Design review of the part built by this model. Coordinates are the model's own, in mm. A direction names the side the tool comes from. Coordinates: 2 decimals unless noted, no trailing zeros. Write each loop counter-clockwise with the first axis right and the second up, starting at its lowest first coordinate (ties: lowest second). Pieces come first, ordered by that corner, then holes. Notation, with made-up numbers: (52, 75.5) - (107, 75.5) arc R21 cw to (107, 109.5) - close; hole circle Ø11 at (-16, 52). An arc over 180 degrees is marked (long way). Answer as CSV lines item,"result". Start each with the question number.
Q1. Machinability: for faces 1 (the face through (0.54, -8.88, -11.56)), 2 (the face through (0.75, -66, 0)), 3 (the face through (4, -70, 0)), 4 (the face through (-1, -42, -12)), 5 (the face through (0, -20, 19)), which of the approach directions +Z, -Z, +X, -X, +Y, -Y give a long, thin tool a straight path to every point of the face, cutting with its end or side? Answer none if there is none.
Q2. We need section C-C (y = -51.5). Write out the cut boundary in (x, z).
Q3. For line 1 along Z through (x, y) = (0, -12.5); line 2 along X through (y, z) = (-4.75, 14); line 3 along Z through (x, y) = (0.5, -12.5), list the stretches that pass through material, from the lowest coordinate up. Write a range as [from, to].
Q4. Mouldability with a two-part tool opening along X and no side actions: class faces 6 (the face through (-1, -42, 12)), 7 (the face through (1.65, -69.14, -0.17)), 8 (the face through (0.23, -18.24, -14.37)) as pulls with the +X half, pulls with the -X half, needs draft (parallel to the pull), parting line crosses it, or undercut.
Q5. We need section A-A (y = -15). Write out the cut boundary in (x, z), plus the area to 3 significant figures.
Q6. Clearance check with flat-ended pins moving along their axes: pin 1 (1 mm diameter, centred on x = 4, z = 3.5, fed in from +Y); pin 2 (6 mm diameter, centred on x = 0, z = 14, fed in from -Y); pin 3 (5.5 mm diameter, centred on x = -0.5, z = -20, fed in from -Y); pin 4 (0.6 mm diameter, centred on y = -66.5, z = -2, fed in from -X). State where each tip first meets the part, or that it passes through.
Q7. We need section D-D (y = -62). Write out the cut boundary in (x, z).
Q8. We need section B-B (z = 8.5). Write out the cut boundary in (x, y).
from build123d import *

# Parameters (mm, degrees)
SKETCH1_W                   = 10.5
SKETCH1_H                   = 24
BOSS_EXTRUDE1_DEPTH         = 70
CUT_EXTRUDE1_REACH          = 76.186
FILLET1_R                   = 3
SKETCH3_W                   = 10.5
SKETCH3_H                   = 44
BOSS_EXTRUDE2_DEPTH         = 20
FILLET2_R                   = 1
M6_TAPPED_HOLE1_D           = 5
M6_TAPPED_HOLE1_DEPTH       = 17
M6_TAPPED_HOLE1_CSINK_D     = 6.05
M6_TAPPED_HOLE1_CSINK_ANGLE = 90
M6_TAPPED_HOLE1_TIP         = 1.502151548
FILLET3_R                   = 5
FILLET4_R                   = 1


with BuildPart() as part:
    # Sketch1 → Boss-Extrude1 (new body)
    with BuildSketch(Plane(origin=(0, 0, 0), x_dir=(1, 0, 0), z_dir=(0, 1, 0))):
        Rectangle(SKETCH1_W, SKETCH1_H)
    extrude(amount=-BOSS_EXTRUDE1_DEPTH)

    # Sketch2 → Cut-Extrude1 (cut, up to next)
    with BuildSketch(Plane.XY.offset(12), mode=Mode.PRIVATE) as cut_extrude1_sk1:
        with BuildLine():
            Line((-1.881919427, -61.241229517), (-5.25, -60.015348442))
            Line((-5.25, -60.015348442), (-5.25, -70))
            Line((-5.25, -70), (0.75, -70))
            Line((0.75, -70), (0.75, -65))
            ThreePointArc((0.75, -65), (0.026608177, -62.705694255), (-1.881919427, -61.241229517))
        make_face()
    cut_extrude1_tool1 = extrude(cut_extrude1_sk1.sketch, amount=-CUT_EXTRUDE1_REACH, mode=Mode.PRIVATE) & part.part
    add(cut_extrude1_tool1.solids().sort_by_distance((-2.443278, -65.612177, 12))[0], mode=Mode.SUBTRACT)

    # Fillet1
    fillet1_edges = [part.edges().sort_by_distance(p)[0] for p in [
        (0.75, -70, 0),
    ]]
    fillet(fillet1_edges, radius=FILLET1_R)

    # Sketch3 → Boss-Extrude2 (add)
    with BuildSketch(Plane(origin=(0, 0, 0), x_dir=(1, 0, 0), z_dir=(0, 1, 0))):
        Rectangle(SKETCH3_W, SKETCH3_H)
    extrude(amount=-BOSS_EXTRUDE2_DEPTH)

    # Fillet2
    fillet2_edges = [part.edges().sort_by_distance(p)[0] for p in [
        (5.25, -45, 12),
        (5.25, -45, -12),
    ]]
    fillet(fillet2_edges, radius=FILLET2_R)

    # M6 Tapped Hole1
    with Locations(Plane(origin=(0, 0, 0), x_dir=(1, 0, 0), z_dir=(0, 1, 0))):
        with Locations((0, 14), (0, -14)):
            CounterSinkHole(M6_TAPPED_HOLE1_D / 2, M6_TAPPED_HOLE1_CSINK_D / 2, depth=M6_TAPPED_HOLE1_DEPTH, counter_sink_angle=M6_TAPPED_HOLE1_CSINK_ANGLE)
            with Locations((0, 0, -(M6_TAPPED_HOLE1_DEPTH + M6_TAPPED_HOLE1_TIP / 2))):  # 118° drill point
                Cone(0, M6_TAPPED_HOLE1_D / 2, M6_TAPPED_HOLE1_TIP, mode=Mode.SUBTRACT)

    # Fillet3
    # the kernel refuses this fillet: 5 mm, written as the material it adds along each edge
    with BuildSketch(Plane(origin=(4.25, -20, 12), x_dir=(0, -1, 0), z_dir=(-1, 0, 0)), Plane(origin=(-5.25, -20, -12), x_dir=(0, -1, 0), z_dir=(1, 0, 0))) as fillet3_piece_1:
        with BuildLine():
            CenterArc((FILLET3_R, FILLET3_R), FILLET3_R, 180, 90)
            Line((0, FILLET3_R), (0, 0))
            Line((0, 0), (FILLET3_R, 0))
        make_face()
    extrude(amount=9.5)
    with BuildSketch(Plane(origin=(4.25, -20, -11), x_dir=(0, 0, -1), z_dir=(-1, 0, 0))) as fillet3_piece_2_section:
        with BuildLine():
            CenterArc((1 + FILLET3_R, FILLET3_R), FILLET3_R, 180, 90)
            Line((1, FILLET3_R), (1, 0))
            Line((1, 0), (1 + FILLET3_R, 0))
        make_face()
    fillet3_piece_2 = revolve(axis=Axis((4.25, -20, -11), (0, -1, 0)), revolution_arc=359.64, mode=Mode.PRIVATE)
    fillet3_piece_2 = split(fillet3_piece_2, bisect_by=Plane(origin=(5.25, -21.017365057, -13.137521002), z_dir=(-1, 0, 0)), keep=Keep.TOP, mode=Mode.PRIVATE)
    add(fillet3_piece_2)
    with BuildSketch(Plane(origin=(4.25, -20, 11), x_dir=(0, 0, 1), z_dir=(-1, 0, 0))) as fillet3_piece_3_section:
        with BuildLine():
            CenterArc((1 + FILLET3_R, -FILLET3_R), FILLET3_R, 90, 90)
            Line((1 + FILLET3_R, 0), (1, 0))
            Line((1, 0), (1, -FILLET3_R))
        make_face()
    fillet3_piece_3 = revolve(axis=Axis((4.25, -20, 11), (0, 1, 0)), revolution_arc=359.64, mode=Mode.PRIVATE)
    fillet3_piece_3 = split(fillet3_piece_3, bisect_by=Plane(origin=(5.25, -22.017645533, 11.767475003), z_dir=(-1, 0, 0)), keep=Keep.TOP, mode=Mode.PRIVATE)
    add(fillet3_piece_3)

    # Fillet4
    fillet4_edges = [part.edges().sort_by_distance(p)[0] for p in [
        (-5.25, -10, 22),
        (-5.25, -10, -22),
        (5.25, -10, -22),
        (5.25, -10, 22),
    ]]
    fillet(fillet4_edges, radius=FILLET4_R)


solid = part.part
Results list:
1,face 1,"+Y"
1,face 2,"+Z, -Z, -X, -Y"
1,face 3,"+Z, -Z, +X, -X, -Y"
1,face 4,"-Z, +X, -X, -Y"
1,face 5,"+Z, +X, -X, -Y"
2,outline,"(-5.25, -12) - (4.25, -12) arc R1 ccw to (5.25, -11) - (5.25, 11) arc R1 ccw to (4.25, 12) - (-5.25, 12) - close"
3,line 1,"z = [-22, -16.5], [-11.5, 11.5], [16.5, 22]"
3,line 2,"x = [-5.25, -2.5], [2.5, 5.25]"
3,line 3,"z = [-22, -16.45], [-11.55, 11.55], [16.45, 22]"
4,face 6,"needs draft"
4,face 7,"pulls with the -X half"
4,face 8,"undercut"
5,outline,"(-5.25, -21) arc R1 ccw to (-4.25, -22) - (4.25, -22) arc R1 ccw to (5.25, -21) - (5.25, 21) arc R1 ccw to (4.25, 22) - (-4.25, 22) arc R1 ccw to (-5.25, 21) - close; hole circle Ø5 at (0, -14); hole circle Ø5 at (0, 14)"
5,area,"422 mm2"
6,pin 1,"stops at y = 0"
6,pin 2,"stops at y = -69.59"
6,pin 3,"stops at y = -20"
6,pin 4,"stops at x = 0.75"
7,outline,"(-0.6, -12) - (4.25, -12) arc R1 ccw to (5.25, -11) - (5.25, 11) arc R1 ccw to (4.25, 12) - (-0.6, 12) - close"
8,outline,"(-5.25, -60.02) - (-1.88, -61.24) arc R4 cw to (0.75, -65) - (0.75, -67) arc R3 ccw to (3.75, -70) - (5.25, -70) - (5.25, 0) - (-5.25, 0) - close"
